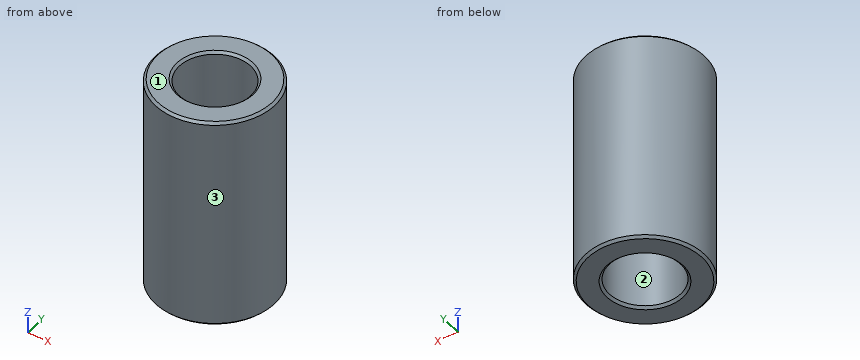
Solid Edge part; units mm, degrees
sketch "Sketch1" plane through (0, 0, 0) normal (0, 0, 1) x (1, 0, 0)
  circle A0 centre (0, 0) radius 12.5
  circle A1 centre (0, 0) radius 7.5
extrude "Extrusionsausprägung_28" add sketch "Sketch1" against normal blind 45
chamfer "Fase_17" distance 0.5 angle 45 2 edges at (-7.5, 0, 0) (-12.5, 0, 0)
chamfer "Fase_18" distance 0.5 angle 45 2 edges at (-7.5, 0, -45) (-12.5, 0, -45)
Design review of the part built by this model. Coordinates are the model's own, in mm. Face numbers are marked on the shaded views. Coordinates: 2 decimals unless noted, no trailing zeros. Write each loop counter-clockwise with the first axis right and the second up, starting at its lowest first coordinate (ties: lowest second). Pieces come first, ordered by that corner, then holes. Notation, with made-up numbers: (-22.75, 87) - (-7.75, 87) arc R26 ccw to (-7.75, 106) - close; hole circle Ø11 at (-36.5, 6). An arc over 180 degrees is marked (long way). Use one line per item in the form item = value.
Q1. The part is to be moulded in two halves that separate along X. For the marked faces 1, 2 and 3, say which applies: +X half, -X half, draft (parallel to the pull), parting line (faces both ways), or undercut.
Taken from the geometry:
face_1 = draft
face_2 = undercut
face_3 = parting line
Q2. For probe 1 along Y at (x, z) = (0, -14); probe 2 along Y at (x, z) = (-4.25, -6.5); probe 3 along Y at (x, z) = (10, -3.5), list the stretches that pass through material, from the lowest coordinate up.
Taken from the geometry:
probe_1 = -12.5 to -7.5, 7.5 to 12.5
probe_2 = -11.76 to -6.18, 6.18 to 11.76
probe_3 = -7.5 to 7.5
Q3. Consider section C-C (z = -15). Write out the cut boundary in (x, y), plus the area to 3 significant figures.
Taken from the geometry:
outline = circle Ø25 at (0, 0); hole circle Ø15 at (0, 0)
area = 314 mm^2
Q4. Consider section A-A (x = 0). Write out the cut boundary in (y, z), plus the area to 3 significant figures.
Taken from the geometry:
outline = (-12.5, -44.5) - (-12, -45) - (-8, -45) - (-7.5, -44.5) - (-7.5, -0.5) - (-8, 0) - (-12, 0) - (-12.5, -0.5) - close; (7.5, -44.5) - (8, -45) - (12, -45) - (12.5, -44.5) - (12.5, -0.5) - (12, 0) - (8, 0) - (7.5, -0.5) - close
area = 449 mm^2
Q5. Insertion check: pin 1 Ø1 at (x, z) = (-6, -34) entering from -Y (3 decimals); pin 2 Ø1.5 at (y, z) = (8.5, -22.5) entering from -X; pin 3 Ø1 at (x, z) = (1, -23) entering from +Y. Each pin has a flat end and moves straight along its axis. Give the tip position at first contact, or say it passes through.
Taken from the geometry:
pin_1 = -11.225
pin_2 = -9.81
pin_3 = 12.49
